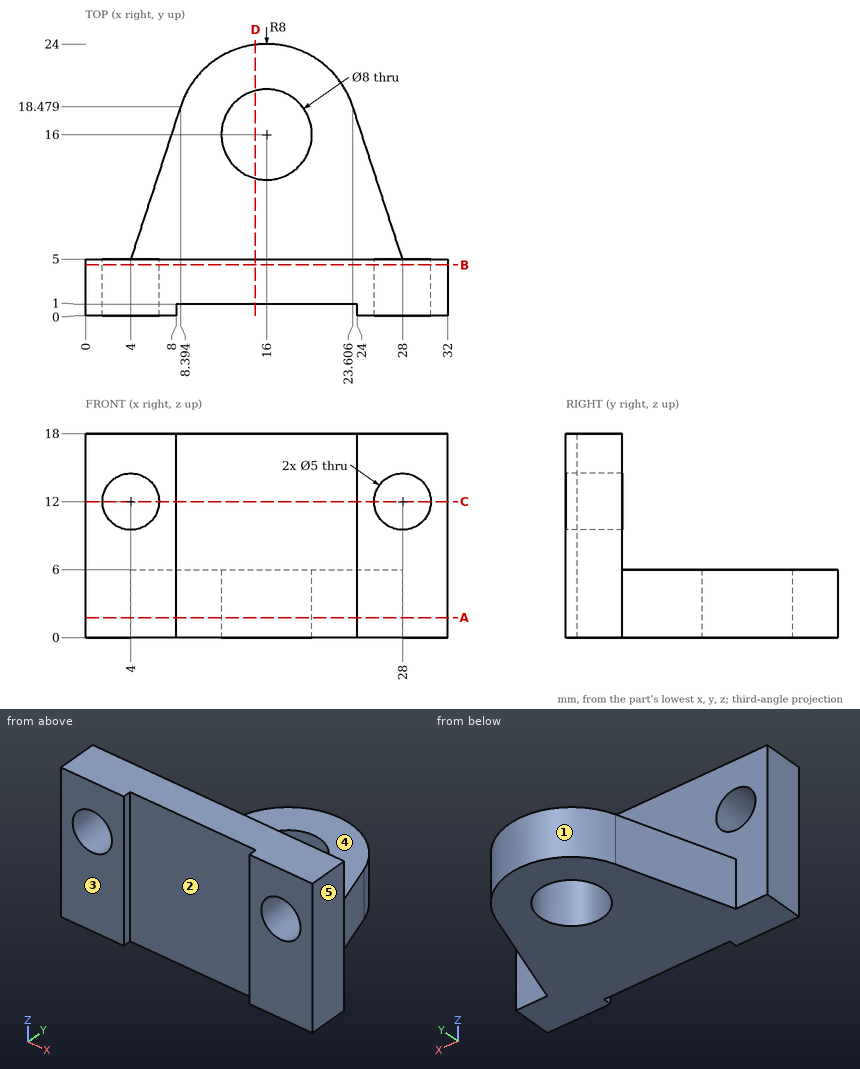
The drawing under review shows one solid part. Ordinate dimensions are in mm from its lowest x, y, z. A direction names the side the tool comes from. Coordinates: 2 decimals unless noted, no trailing zeros. Order: outer loops, then holes, each group sorted by start corner. A loop starts at its lowest first (then second) coordinate and runs counter-clockwise, first axis right, second up. Notation, with made-up numbers: (15, -33) -> (48, -33) arc R21 cw to (48, -6) -> close; hole circle Ø6 at (-30, 78.25). An arc over 180 degrees is marked (long way). One line per item, written item: value.
1) We need section D-D, the plane x = 15. Give the boundary of the cut face in (y, z).
Output values:
outline: (1, 0) -> (12.13, 0) -> (12.13, 6) -> (5, 6) -> (5, 18) -> (1, 18) -> close; (19.87, 0) -> (23.94, 0) -> (23.94, 6) -> (19.87, 6) -> close
2) We need section A-A, the plane z = 1.75. Give the boundary of the cut face in (x, y).
Output values:
outline: (0, 0) -> (8, 0) -> (8, 1) -> (24, 1) -> (24, 0) -> (32, 0) -> (32, 5) -> (28, 5) -> (23.61, 18.48) arc R8 ccw to (8.39, 18.48) -> (4, 5) -> (0, 5) -> close; hole circle Ø8 at (16, 16)
3) Clearance check with flat-ended pins moving along their axes: P1, Ø3, axis at x = 25, y = 8.5, coming from the +Z side; P2, Ø5, axis at x = 14, z = 12, coming from the -Y side; P3, Ø6.5, axis at x = 28, z = 12, coming from the +Y side. State where each tip first meets the part, or that it passes through.
Output values:
P1: stops at z = 6
P2: stops at y = 1
P3: stops at y = 5
4) We need section B-B, the plane y = 4.5. Give the boundary of the cut face in (x, z).
Output values:
outline: (0, 0) -> (32, 0) -> (32, 18) -> (0, 18) -> close; hole circle Ø5 at (4, 12); hole circle Ø5 at (28, 12)
5) We need section C-C, the plane z = 12. Give the boundary of the cut face in (x, y).
Output values:
outline: (0, 0) -> (1.5, 0) -> (1.5, 5) -> (0, 5) -> close; (6.5, 0) -> (8, 0) -> (8, 1) -> (24, 1) -> (24, 0) -> (25.5, 0) -> (25.5, 5) -> (6.5, 5) -> close; (30.5, 0) -> (32, 0) -> (32, 5) -> (30.5, 5) -> close
6) Draft analysis for pull direction X (two halves, no side actions). For the marked faces 1, 2 and 3, state which applies: +X half, -X half, draft (parallel to the pull), parting line (faces both ways), or undercut.
Output values:
face 1: parting line
face 2: undercut
face 3: draft
7) To check wall thickness, follow probe 1 along X at (y, z) = (2.55, 12); probe 2 along Z at (x, y) = (28, 1.05); probe 3 along Y at (x, z) = (14.5, 16.25). State the ranges of each line that lie inside material, in increasing order. Write a range as [from, to].
Output values:
probe 1: x = [0, 1.5], [6.5, 25.5], [30.5, 32]
probe 2: z = [0, 9.5], [14.5, 18]
probe 3: y = [1, 5]
8) Machinability: for the marked faces 4 and 5, which of the approach directions +Z, -Z, +X, -X, +Y, -Y give a long, thin tool a straight path to every point of the face, cutting with its end or side? Answer none if there is none.
Output values:
face 4: +Z, +X, -X, +Y
face 5: +Z, -Z, +X, +Y, -Y
